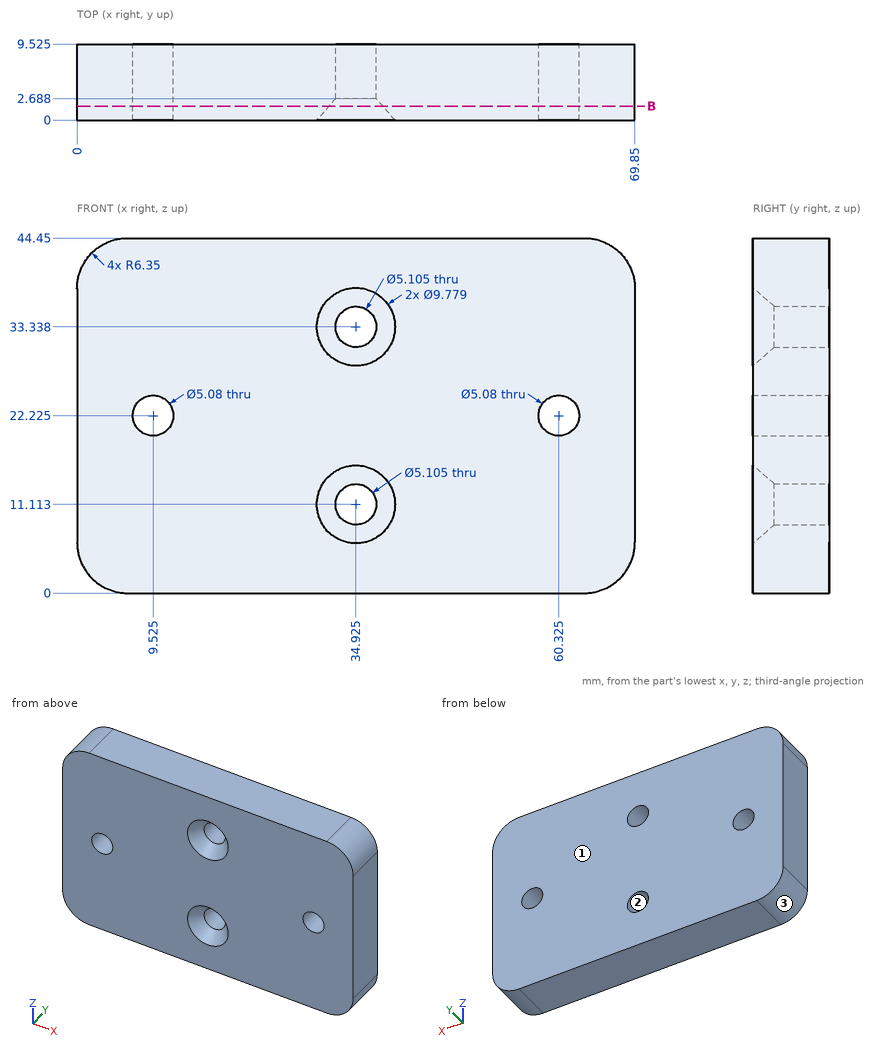
Geometry check sheet. Reference: drawing and pictorial views, mm from the part's lowest x, y, z. Give positions to 0.01 mm unless a question says otherwise; leave off trailing zeros. Put each result on its own line as item: value. Start each with the question number.
1. Scan lines: line 1 along X through (y, z) = (8, 22.5); line 2 along X through (y, z) = (2, 21); line 3 along X through (y, z) = (8, 38.5). Record each from-to range of solid material in increasing order. Write a range as [from, to].
2. Draft check along Z on the marked faces 1, 2 and 3. Enter one of: +Z half, -Z half, draft (parallel to the pull), parting line (faces both ways), or undercut.
3. Section check B-B (y = 1.75). Give the number of separate pieces and of enclosed holes in the cut face, and give its area (3 significant figures).
4. Go/stop test with a flat-tipped pin: pin 1 Ø4 at (x, z) = (34.92, 11.11) entering from -Y. Record where the tip stops, or that it passes through.
Answer list:
1. line 1: [0, 7], [12.05, 57.8], [62.85, 69.85]
1. line 2: [0, 7.3], [11.75, 58.1], [62.55, 69.85]
1. line 3: [0.01, 69.84]
2. face 1: draft
2. face 2: undercut
2. face 3: -Z half
3. separate pieces: 1
3. enclosed holes: 4
3. area: 2,960 mm2
4. pin 1: through
